Here's how the part is built. I have some questions about the finished solid (model axes, mm). Give positions to 0.01 mm unless a question says otherwise; leave off trailing zeros. Order: outer loops, then holes, each group sorted by start corner. A loop starts at its lowest first (then second) coordinate and runs counter-clockwise, first axis right, second up.
Autodesk Fusion 360 part; units mm, degrees
sketch "Sketch1" plane through (0, 0, 0) normal (0, 0, 1) x (1, 0, 0)
  circle A0 centre (0, 0) radius 6
  circle A1 centre (0, 0) radius 7.5
  circle A2 centre (0, 0) radius 5.15
  dimension "d1" = 12
  dimension "d2" = 15
  dimension "d3" = 10.3
extrude "Extrude1" add sketch "Sketch1" along normal blind 4.2 contours A0 | A1
chamfer "Chamfer1" distance 0.8 distance2 4.2 1 edges at (-4.8015, 1.8623, 4.2) measured on face at (6.6696, -0.6285, 4.2)
extrude "Extrude2" add sketch "Sketch1" against normal blind 3 contours A0 | A1 | A2
Q1. I need wall thicknesses on L1, parallel to Z at x = 2, y = 2.25; L2, parallel to X at y = 2, z = 1; L3, parallel to X at y = -4.75, z = 0.25. Which ranges of each line are inside material? Lowest first, please.
Filled sheet:
L1: z = -3 to 0
L2: x = -7.23 to -4.95, 4.95 to 7.23
L3: x = -5.8 to -2.11, 2.11 to 5.8
Q2. Thinking about a two-plate mould opening in X: for faces 1 (the face through (0, 0, -3)), 2 (the face through (5.13, 1.62, 1.2)), 3 (the face through (0, 0, 0)), 4 (the face through (-7.493, -0.33, 0.55)), which applies, released by +X, released by -X, zero draft, split by the parting line, or undercut?
Filled sheet:
face 1: zero draft
face 2: undercut
face 3: undercut
face 4: split by the parting line
Q3. If we section it at D-D on z = 2.5: List the corners of the cut face in (x, y) for me.
Filled sheet:
outline: circle Ø15 at (0, 0); hole circle Ø11.25 at (0, 0)
Q4. I'm going to push flat-ended pins straight in: P1, Ø4, axis at x = 0.5, z = 2, coming from the -Y side; P2, Ø1, axis at y = 5, z = 0, coming from the +X side; P3, Ø1, axis at x = 2, y = -3, coming from the +Z side. Where does each tip first touch, or does it pass through?
Filled sheet:
P1: stops at y = -7.5
P2: stops at x = 6
P3: stops at z = 0
Q5. If we section it at C-C on z = -2: List the corners of the cut face in (x, y) for me.
Filled sheet:
outline: circle Ø15 at (0, 0)
